```python
from build123d import *

# Parameters (mm, degrees)
F1_DEPTH = 8.89
F2_T     = -1.27
F3_D     = 1.778


# Not quite as in the source:
# - a feature names something its author has since deleted; it is built from what else it names


with BuildPart() as f1:
    # F0 (on Front) → F1 (new body)
    with BuildSketch(Plane.XZ):
        Polygon((-45.8687357605, 33.5707478225), (-45.5147512257, 46.3788583875), (-53.0798770487, 46.3788583875), (-53.0798770487, 30.4408613592), align=None)
    extrude(amount=F1_DEPTH)

    # F2
    f2_openings = [f1.faces().sort_by_distance(p)[0] for p in [
        (-49.297314, -4.445, 46.378858),
        (-53.079877, -4.445, 38.40986),
        (-49.474306, -4.445, 32.005805),
    ]]
    offset(amount=F2_T, openings=f2_openings)

    # F3 (through all)
    with Locations(Plane(origin=(0, 0, 0), x_dir=(1, 0, 0), z_dir=(0, 1, 0))):
        with Locations((-49.2973141372, -43.3367788792), (-49.3943579495, -34.0744107962)):
            Hole(F3_D / 2)


solid = f1.part
```
The listing builds one solid part. Answer for the finished solid, in the listing's coordinates (mm). Give positions to 0.01 mm unless a question says otherwise; leave off trailing zeros. Order: outer loops, then holes, each group sorted by start corner. A loop starts at its lowest first (then second) coordinate and runs counter-clockwise, first axis right, second up. Notation, with made-up numbers: (83.5, 62) -> (125.5, 62) arc R24 cw to (125.5, 79) -> close; hole circle Ø9 at (-25, 55). An arc over 180 degrees is marked (long way). One line per item, written item: value.
1) Find section A-A, the plane x = -48.25. Determine the outline of the cut face in (y, z).
Reported:
outline: (-8.89, 32.54) -> (-7.62, 32.54) -> (-7.62, 46.38) -> (-8.89, 46.38) -> close; (-1.27, 32.54) -> (0, 32.54) -> (0, 46.38) -> (-1.27, 46.38) -> close
2) Determine the mould class of faces 1 (the flat face through (-46, -4, 46.379)), 2 (the cylindrical face through (-48.69, -0.64, 34.62)), 3 (the cylindrical face through (-49.78, -8.26, 42.59)), 4 (the flat face through (-53.08, -1, 39)) for opening direction X: pulls with the +X half, pulls with the -X half, needs draft (parallel to the pull), parting line crosses it, or undercut.
Reported:
face 1: needs draft
face 2: undercut
face 3: undercut
face 4: pulls with the -X half
3) Find section C-C, the plane x = -49.25. Determine the outline of the cut face in (y, z), plus the area to 3 significant figures.
Reported:
outline: (-8.89, 32.1) -> (-7.62, 32.1) -> (-7.62, 33.2) -> (-8.89, 33.2) -> close; (-8.89, 34.95) -> (-7.62, 34.95) -> (-7.62, 42.45) -> (-8.89, 42.45) -> close; (-8.89, 44.22) -> (-7.62, 44.22) -> (-7.62, 46.38) -> (-8.89, 46.38) -> close; (-1.27, 32.1) -> (0, 32.1) -> (0, 33.2) -> (-1.27, 33.2) -> close; (-1.27, 34.95) -> (0, 34.95) -> (0, 42.45) -> (-1.27, 42.45) -> close; (-1.27, 44.22) -> (0, 44.22) -> (0, 46.38) -> (-1.27, 46.38) -> close
area: 27.3 mm^2
4) Find the intervals of material crossed by line 1 (Y direction, x = -48, z = 34.75); line 2 (Z direction, x = -49.25, y = -8); line 3 (Z direction, x = -51.5, y = -0.25), in increasing order.
Reported:
line 1: y = -8.89 to -7.62, -1.27 to 0
line 2: z = 32.1 to 33.2, 34.95 to 42.45, 44.22 to 46.38
line 3: z = 31.13 to 46.38
5) Find section D-D, the plane z = 37. Determine the outline of the cut face in (x, y), plus the area to 3 significant figures.
Reported:
outline: (-53.08, -8.89) -> (-45.77, -8.89) -> (-45.77, 0) -> (-53.08, 0) -> (-53.08, -1.27) -> (-47.04, -1.27) -> (-47.04, -7.62) -> (-53.08, -7.62) -> close
area: 26.6 mm^2
6) Flat-ended cylindrical pins translate along their axes: P1, Ø2, axis at y = -4.5, z = 35, coming from the -X side; P2, Ø4, axis at x = -48, y = -3.5, coming from the -Z side; P3, Ø2, axis at x = -49.39, z = 34.07, coming from the -Y side. Find the tip coordinate at first contact, or state that the pin passes through.
Reported:
P1: stops at x = -47.13
P2: stops at z = 33.01
P3: stops at y = -8.89
7) Find section B-B, the plane z = 34.75. Determine the outline of the cut face in (x, y).
Reported:
outline: (-53.08, -8.89) -> (-49.97, -8.89) -> (-49.97, -7.62) -> (-53.08, -7.62) -> close; (-53.08, -1.27) -> (-49.97, -1.27) -> (-49.97, 0) -> (-53.08, 0) -> close; (-48.82, -8.89) -> (-45.84, -8.89) -> (-45.84, 0) -> (-48.82, 0) -> (-48.82, -1.27) -> (-47.11, -1.27) -> (-47.11, -7.62) -> (-48.82, -7.62) -> close
